Read the model definition and answer for the solid it produces. Units are mm, in the model's axes. Face numbers are marked on the shaded views. Round coordinates to 2 decimals unless told otherwise and drop trailing zeros. Order: outer loops, then holes, each group sorted by start corner. A loop starts at its lowest first (then second) coordinate and runs counter-clockwise, first axis right, second up.
from build123d import *

# Parameters (mm, degrees)
F2_W     = 200
F2_H     = 10
F3_DEPTH = 125
F4_R     = 7.5
F5_DEPTH = 100
F6_R     = 4.5
F7_DEPTH = 6
F8_R     = 4.2
F9_DEPTH = 5


with BuildPart() as f3:
    # F2 (on Right) → F3 (new body, symmetric)
    with BuildSketch(Plane.YZ):
        with Locations((0, 5)):
            Rectangle(F2_W, F2_H)
    extrude(amount=F3_DEPTH, both=True)

    # F4 (on face) → F5 (join)
    with BuildSketch(Plane(origin=(0, 0, 0), x_dir=(1, 0, 0), z_dir=(0, 0, -1))):
        with Locations((-117.5, -92.5)):
            Circle(F4_R)
        with Locations((117.5, -92.5)):
            Circle(F4_R)
        with Locations((117.5, 92.5)):
            Circle(F4_R)
        with Locations((-117.5, 92.5)):
            Circle(F4_R)
    extrude(amount=-F5_DEPTH)

    # F6 (on face) → F7 (cut)
    with BuildSketch(Plane(origin=(0, 0, 0), x_dir=(1, 0, 0), z_dir=(0, 0, -1))):
        with Locations((-117.5, 92.5)):
            Circle(F6_R)
        with Locations((-117.5, -92.5)):
            Circle(F6_R)
        with Locations((117.5, 92.5)):
            Circle(F6_R)
        with Locations((117.5, -92.5)):
            Circle(F6_R)
    extrude(amount=-F7_DEPTH, mode=Mode.SUBTRACT)

    # F8 (on face) → F9 (join)
    with BuildSketch(Plane.XY.offset(100)):
        with Locations((-117.5, 92.5)):
            Circle(F8_R)
        with Locations((117.5, 92.5)):
            Circle(F8_R)
        with Locations((117.5, -92.5)):
            Circle(F8_R)
        with Locations((-117.5, -92.5)):
            Circle(F8_R)
    extrude(amount=F9_DEPTH)


solid = f3.part
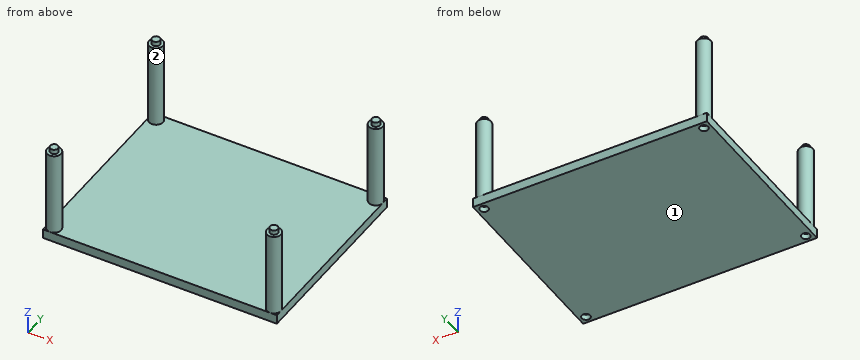
Q1. A cutting plane is placed at C-C, the plane y = -21.5. Give the vertices of the cut face in (x, z).
Outcome:
outline: (-125, 0) - (125, 0) - (125, 10) - (-125, 10) - close
Q2. A cutting plane is placed at B-B, the plane x = 14. Give the vertices of the cut face in (y, z), plus the area to 3 significant figures.
Outcome:
outline: (-100, 0) - (100, 0) - (100, 10) - (-100, 10) - close
area: 2,000 mm2
Q3. For a pull along X with two mould halves and no side action, classify the marked faces 1 and 2 as released by +X, released by -X, zero draft, split by the parting line, or undercut.
Outcome:
face 1: zero draft
face 2: undercut
Q4. A flat-ended cylindrical pin translates along its axis: pin 1 (4.5 mm diameter, centred on x = -121, y = 90, fed in from +Z). Find the tip coordinate at first contact, or state that the pin passes through.
Outcome:
pin 1: stops at z = 105
Q5. A cutting plane is placed at A-A, the plane z = 71.5. Give the vertices of the cut face in (x, y).
Outcome:
outline: circle Ø15 at (-117.5, -92.5); circle Ø15 at (-117.5, 92.5); circle Ø15 at (117.5, -92.5); circle Ø15 at (117.5, 92.5)
Q6. Straight lines are drawn through the part: probe 1 along X at (y, z) = (-92.5, 3.6); probe 2 along Y at (x, z) = (117.5, 3.35); probe 3 along Z at (x, y) = (-56, 55.5). For each, find the intervals that lie inside material, in ascending order.
Outcome:
probe 1: x = -125 to -122, -113 to 113, 122 to 125
probe 2: y = -100 to -97, -88 to 88, 97 to 100
probe 3: z = 0 to 10
